```python
from build123d import *

# Parameters (mm, degrees)
EXTRUDE_1_DEPTH     = 45
SKETCH_2_R          = 20
CUT_EXTRUDE_1_DEPTH = 20
SKETCH_3_W          = 5
SKETCH_3_H          = 6.5
CUT_EXTRUDE_2_DEPTH = 20
SKETCH_4_W          = 5
SKETCH_4_H          = 6.5
CUT_EXTRUDE_3_DEPTH = 20


with BuildPart() as part:
    # Эскиз1 → Бобышка-Вытянуть1 (new body)
    with BuildSketch(Plane(origin=(0, 0, 0), x_dir=(0, 0, -1), z_dir=(1, 0, 0))):
        Polygon((0, 0), (0, 40), (15, 40), (15, 48.5), (16, 48.5), (16, 62.5), (60, 62.5), (60, 48.5), (61, 48.5), (61, 40), (76, 40), (76, 0), (56, 0), (56, 5), (20, 5), (20, 3), (22, 0), align=None)
    extrude(amount=EXTRUDE_1_DEPTH)

    # Эскиз2 → Вырез-Вытянуть1 (cut)
    with BuildSketch(Plane(origin=(0, 62.5, 0), x_dir=(1, 0, 0), z_dir=(0, 1, 0))):
        with Locations((22.5, 38.5)):
            Circle(SKETCH_2_R)
    extrude(amount=-CUT_EXTRUDE_1_DEPTH, mode=Mode.SUBTRACT)

    # Эскиз3 → Вырез-Вытянуть2 (cut)
    with BuildSketch(Plane.XY):
        with Locations((32.5, 17.75)):
            Rectangle(SKETCH_3_W, SKETCH_3_H)
    extrude(amount=-CUT_EXTRUDE_2_DEPTH, mode=Mode.SUBTRACT)

    # Эскиз4 → Вырез-Вытянуть3 (cut)
    with BuildSketch(Plane(origin=(0, 0, -76), x_dir=(-1, 0, 0), z_dir=(0, 0, -1))):
        with Locations((-32.5, 17.75)):
            Rectangle(SKETCH_4_W, SKETCH_4_H)
        with Locations((-12.5, 17.75)):
            Rectangle(SKETCH_4_W, SKETCH_4_H)
    extrude(amount=-CUT_EXTRUDE_3_DEPTH, mode=Mode.SUBTRACT)


solid = part.part
```
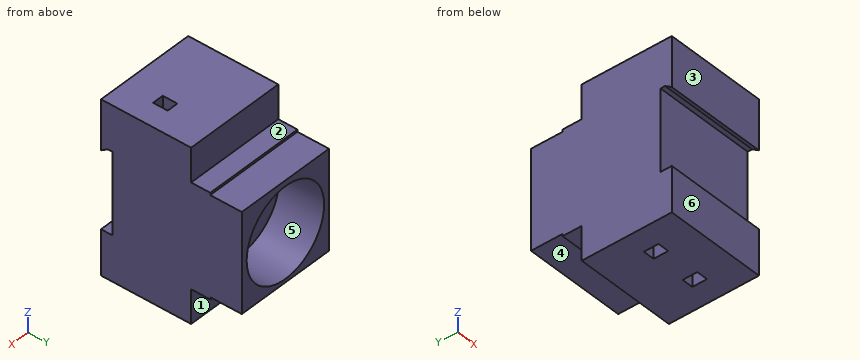
Input: part model. Units: mm. Frame: model coordinates. Face numbers are marked on the shaded views. A direction names the side the tool comes from. Give positions to 0.01 mm unless a question says otherwise; leave off trailing zeros. Order: outer loops, then holes, each group sorted by start corner. A loop starts at its lowest first (then second) coordinate and runs counter-clockwise, first axis right, second up. Notation, with made-up numbers: (-20.75, 48.25) - (13.25, 48.25) arc R16 ccw to (13.25, 75.25) - close; hole circle Ø7 at (33, 12.25). An arc over 180 degrees is marked (long way). Use a Markdown table: item, result.
(1) Pin query (flat end, axial travel): pin 1 (11 mm diameter, centred on x = 13, y = 56.5, fed in from +Z); pin 2 (7 mm diameter, centred on x = 25, y = 54, fed in from -Z); pin 3 (6 mm diameter, centred on x = 14, z = -45.5, fed in from +Y). Return the tip coordinate at first contact, or that it passes through.
Computed values:
| item | result |
|---|---|
| pin 1 | stops at z = -16 |
| pin 2 | stops at z = -60 |
| pin 3 | stops at y = 42.5 |
(2) Section query B-B (y = 51.5). Output: boundary loops of the cut face in (x, z), then the cut area to 3 significant figures.
Computed values:
| item | result |
|---|---|
| outline | (0, -60) - (45, -60) - (45, -16) - (0, -16) - close; hole circle Ø40 at (22.5, -38.5) |
| area | 723 mm2 |
(3) Access query for the marked faces 1, 2 and 3. Directions: +Z, -Z, +X, -X, +Y, -Y. A direction counts if a zero-diameter tool reaches every point of the face in a straight line with its end or side. Return the directions, or none.
Computed values:
| item | result |
|---|---|
| face 1 | -Z, +X, -X, +Y |
| face 2 | +Z, +X, -X, +Y |
| face 3 | +Z, -Z, +X, -X, -Y |
(4) Section query C-C (z = -38.5). Output: boundary loops of the cut face in (x, y), then the cut area to 3 significant figures.
Computed values:
| item | result |
|---|---|
| outline | (0, 5) - (45, 5) - (45, 62.5) - (42.5, 62.5) - (42.5, 42.5) - (2.5, 42.5) - (2.5, 62.5) - (0, 62.5) - close |
| area | 1,790 mm2 |
(5) Section query A-A (x = 22.5). Output: boundary loops of the cut face in (y, z).
Computed values:
| item | result |
|---|---|
| outline | (0, -76) - (40, -76) - (40, -61) - (48.5, -61) - (48.5, -60) - (62.5, -60) - (62.5, -58.5) - (42.5, -58.5) - (42.5, -18.5) - (62.5, -18.5) - (62.5, -16) - (48.5, -16) - (48.5, -15) - (40, -15) - (40, 0) - (0, 0) - (0, -22) - (3, -20) - (5, -20) - (5, -56) - (0, -56) - close |
(6) Draft query along Z for the marked faces 4, 5 and 6. Return one class per face: released by +Z, released by -Z, zero draft, split by the parting line, or undercut.
Computed values:
| item | result |
|---|---|
| face 4 | released by -Z |
| face 5 | undercut |
| face 6 | zero draft |
(7) Section query D-D (x = 6). Output: boundary loops of the cut face in (y, z), then the cut area to 3 significant figures.
Computed values:
| item | result |
|---|---|
| outline | (0, -76) - (40, -76) - (40, -61) - (48.5, -61) - (48.5, -60) - (62.5, -60) - (62.5, -49.8) - (42.5, -49.8) - (42.5, -27.2) - (62.5, -27.2) - (62.5, -16) - (48.5, -16) - (48.5, -15) - (40, -15) - (40, 0) - (0, 0) - (0, -22) - (3, -20) - (5, -20) - (5, -56) - (0, -56) - close |
| area | 3,420 mm2 |
(8) Line query: line 1 (X direction, y = 49.5, z = -38.5); line 2 (Z direction, x = 19.5, y = 4); line 3 (Z direction, x = 22.5, y = 56.25). Output: solid intervals per line, ascending. Write a range as from..to.
Computed values:
| item | result |
|---|---|
| line 1 | x = 0..2.5, 42.5..45 |
| line 2 | z = -76..-56, -20..0 |
| line 3 | z = -60..-58.5, -18.5..-16 |
